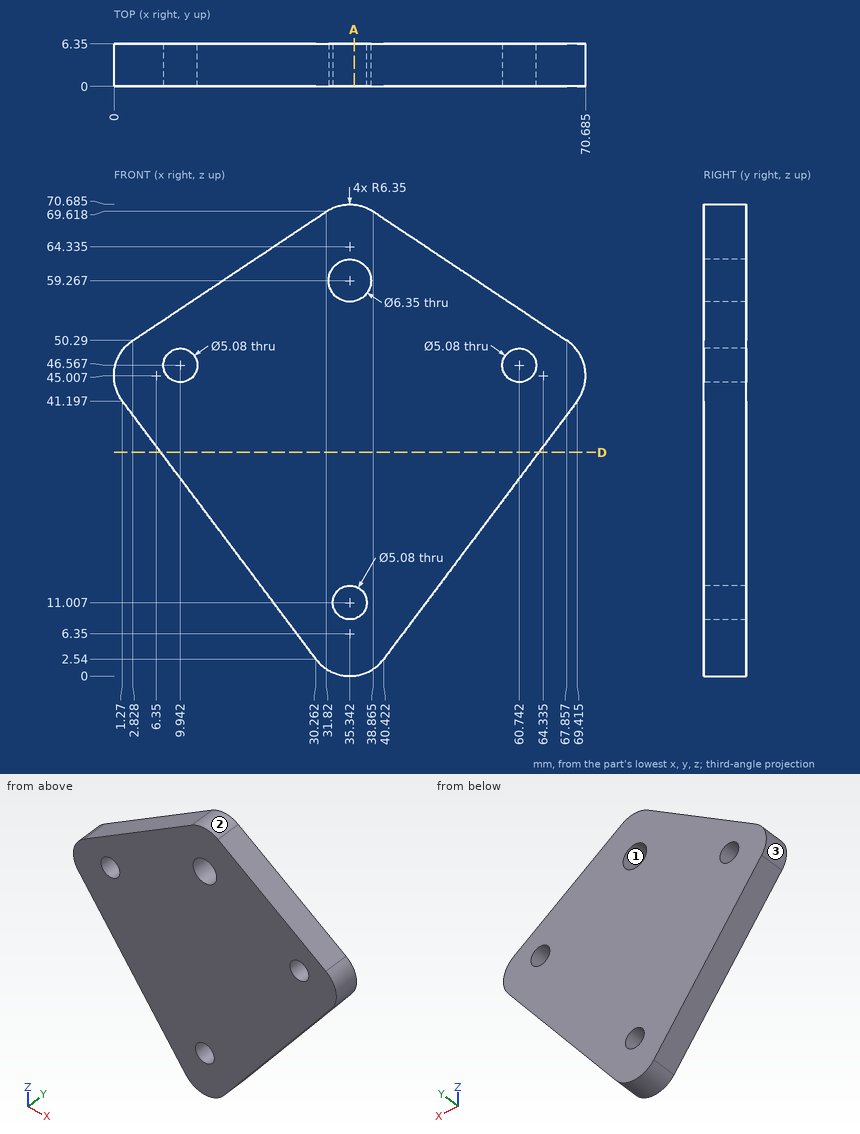
The drawing under review shows one solid part. Ordinate dimensions are in mm from its lowest x, y, z. Coordinates: 2 decimals unless noted, no trailing zeros. Write each loop counter-clockwise with the first axis right and the second up, starting at its lowest first coordinate (ties: lowest second). Pieces come first, ordered by that corner, then holes.
1) Mouldability with a two-part tool opening along X and no side actions: class the marked faces 1, 2 and 3 as +X half, -X half, draft (parallel to the pull), parting line (faces both ways), or undercut.
2) Insertion check: pin 1 (1 mm diameter, centred on y = 0.5, z = 37, fed in from -X); pin 2 (7.5 mm diameter, centred on x = 35.34, z = 59.27, fed in from +Y); pin 3 (1 mm diameter, centred on x = 38, y = 3, fed in from -Z); pin 4 (2 mm diameter, centred on x = 46.5, y = 5.5, fed in from +Z) (1 decimal). Each pin has a flat end and moves straight along its axis. Give the tip position at first contact, or say it passes through.
3) To check wall thickness, follow L1, parallel to Z at x = 61.5, y = 4.5 (1 decimal); L2, parallel to X at y = 2.5, z = 33; L3, parallel to Z at x = 62.5, y = 5.25 (1 decimal). State the ranges of each line that lie inside material, in increasing order.
4) Add section D-D (z = 33.5). Write out the cut boundary in (x, y).
5) Add section A-A (x = 36). State how many separate pieces and enclosed holes the cut face has, plus the area to 3 significant figures.
Check result:
1. face 1: undercut
1. face 2: parting line
1. face 3: -X half
2. pin 1: stops at x = 4.04
2. pin 2: stops at y = 6.35
2. pin 3: stops at z = 0.38
2. pin 4: stops at z = 65.2
3. L1: z = 30.6 to 44.1, 49 to 54.5
3. L2: x = 7.42 to 63.27
3. L3: z = 32 to 44.7, 48.4 to 53.9
4. outline: (7.04, 0) - (63.64, 0) - (63.64, 6.35) - (7.04, 6.35) - close
5. separate pieces: 3
5. enclosed holes: 0
5. area: 378 mm2
